Part model, mm, in its own coordinate system. A direction names the side the tool comes from. Coordinates: 2 decimals unless noted, no trailing zeros. Order: outer loops, then holes, each group sorted by start corner. A loop starts at its lowest first (then second) coordinate and runs counter-clockwise, first axis right, second up.
from build123d import *

# Parameters (mm, degrees)
CROQUIS1_R              = 43.5
SALIENTE_EXTRUIR1_DEPTH = 4
CROQUIS2_R              = 43.5
CROQUIS2_R_2            = 39.017907213
SALIENTE_EXTRUIR2_DEPTH = 2.5
CROQUIS3_R              = 38.31099811
CROQUIS3_R_2            = 33.604332007
SALIENTE_EXTRUIR3_DEPTH = 2.5


with BuildPart() as part:
    # Croquis1 → Saliente-Extruir1 (new body)
    with BuildSketch(Plane(origin=(0, 0, 0), x_dir=(1, 0, 0), z_dir=(0, 1, 0))):
        Circle(CROQUIS1_R)
    extrude(amount=SALIENTE_EXTRUIR1_DEPTH)

    # Croquis2 → Saliente-Extruir2 (add)
    with BuildSketch(Plane(origin=(0, 4, 0), x_dir=(1, 0, 0), z_dir=(0, 1, 0))):
        Circle(CROQUIS2_R)
        Circle(CROQUIS2_R_2, mode=Mode.SUBTRACT)
    extrude(amount=SALIENTE_EXTRUIR2_DEPTH)

    # Croquis3 → Saliente-Extruir3 (add)
    with BuildSketch(Plane.XZ):
        Circle(CROQUIS3_R)
        Circle(CROQUIS3_R_2, mode=Mode.SUBTRACT)
    extrude(amount=SALIENTE_EXTRUIR3_DEPTH)


solid = part.part
Q1. Cut at C-C on y = -1.25. Write the cut outline in (x, z).
Results list:
outline: circle Ø76.62 at (0, 0); hole circle Ø67.21 at (0, 0)
Q2. Pin check, flat tips, straight feed: pin 1 Ø5 at (x, z) = (29, -18.5) entering from +Y; pin 2 Ø1.5 at (x, y) = (17.5, 3.5) entering from -Z; pin 3 Ø3 at (x, y) = (34.5, 0) entering from +Z. Stop position of each tip, or through.
Results list:
pin 1: stops at y = 4
pin 2: stops at z = -40.15
pin 3: stops at z = 28.34
Q3. Wall check: line 1 along Z through (x, y) = (0, 5.8); line 2 along X through (y, z) = (-1, -1). Give the ranges that are in metal, low to high.
Results list:
line 1: z = -43.5 to -39.02, 39.02 to 43.5
line 2: x = -38.3 to -33.59, 33.59 to 38.3
Q4. Cut at A-A on z = 0. Write the cut outline in (x, y), and give its area (3 significant figures).
Results list:
outline: (-43.5, 0) - (-38.31, 0) - (-38.31, -2.5) - (-33.6, -2.5) - (-33.6, 0) - (33.6, 0) - (33.6, -2.5) - (38.31, -2.5) - (38.31, 0) - (43.5, 0) - (43.5, 6.5) - (39.02, 6.5) - (39.02, 4) - (-39.02, 4) - (-39.02, 6.5) - (-43.5, 6.5) - close
area: 394 mm2
Q5. Cut at D-D on z = -35.5. Write the cut outline in (x, y), and give its area (3 significant figures).
Results list:
outline: (-25.14, 0) - (-14.4, 0) - (-14.4, -2.5) - (14.4, -2.5) - (14.4, 0) - (25.14, 0) - (25.14, 6.5) - (16.19, 6.5) - (16.19, 4) - (-16.19, 4) - (-16.19, 6.5) - (-25.14, 6.5) - close
area: 318 mm2
Q6. Mould opens along Z. For faces 4 (the face through (0, 0, 0)), 5 (the face through (0, -2.5, -34)), 6 (the face through (-1, 4, -1)), 7 (the face through (-5.66, 3.2, -43.13)) say: pulls with the +Z half, pulls with the -Z half, needs draft (parallel to the pull), parting line crosses it, or undercut.
Results list:
face 4: undercut
face 5: needs draft
face 6: undercut
face 7: parting line crosses it
Q7. Cut at B-B on x = 0. Write the cut outline in (y, z), and give its area (3 significant figures).
Results list:
outline: (-2.5, -38.31) - (0, -38.31) - (0, -43.5) - (6.5, -43.5) - (6.5, -39.02) - (4, -39.02) - (4, 39.02) - (6.5, 39.02) - (6.5, 43.5) - (0, 43.5) - (0, 38.31) - (-2.5, 38.31) - (-2.5, 33.6) - (0, 33.6) - (0, -33.6) - (-2.5, -33.6) - close
area: 394 mm2
Q8. Which spindle directions (+Z, -Z, +X, -X, +Y, -Y) get a long thin tool onto all of the face, cutting with end or side? Do faces 1 (the face through (-16, 6.5, -36)), 2 (the face through (-8.46, 5.23, 38.09)), 3 (the face through (-4.37, -1.23, 33.32)). Say none if no direction does.
Results list:
face 1: +Z, -Z, +X, -X, +Y
face 2: +Y
face 3: -Y
